```python
from build123d import *

# Parameters (mm, degrees)
F0_W     = 101.6
F0_H     = 101.6
F1_DEPTH = 6.35
F2_R     = 3.175
F3_DEPTH = 6.351
F4_W     = 6.35
F4_H     = 50.8
F5_DEPTH = 6.351


with BuildPart() as f1:
    # F0 (on Top) → F1 (new body)
    with BuildSketch(Plane.XY):
        Rectangle(F0_W, F0_H)
    extrude(amount=F1_DEPTH)

    # F2 (on Top) → F3 (cut, through all)
    with BuildSketch(Plane.XY):
        with Locations((-6.35, 0)):
            Circle(F2_R)
    extrude(amount=F3_DEPTH, mode=Mode.SUBTRACT)

    # F4 (on Top) → F5 (cut, through all)
    with BuildSketch(Plane.XY):
        with Locations((-41.275, 25.4)):
            Rectangle(F4_W, F4_H)
    extrude(amount=F5_DEPTH, mode=Mode.SUBTRACT)


solid = f1.part
```
Source: CAD feature listing. Evaluate the final solid. Frame: model axes, mm. A direction names the side the tool comes from. Round coordinates to 2 decimals unless told otherwise and drop trailing zeros. Loops run counter-clockwise (first coordinate to the right, second up) from the corner with the lowest first, then second, coordinate; pieces in that order, holes last.
1. Section query B-B on x = -6.35. Output: boundary loops of the cut face in (y, z) (3 decimals).
2. Ray query, L1, parallel to X at y = 43, z = 1.75; L2, parallel to Y at x = -6.35, z = 3 (3 decimals); L3, parallel to Y at x = -38.5, z = 3. Return the intervals inside material, ascending.
3. Section query C-C on z = 4.75. Output: boundary loops of the cut face in (x, y) (3 decimals).
4. Access query for faces 4 (the cylindrical face through (-3.32, 0.95, 3.13)), 5 (the flat face through (-41, 0, 3)). Directions: +Z, -Z, +X, -X, +Y, -Y. A direction counts if a zero-diameter tool reaches every point of the face in a straight line with its end or side. Return the directions, or none.
5. Contact query for a flat-ended pin moving along its axis: pin 1 (3 mm diameter, centred on x = -42, z = 4, fed in from +Y). Output: stop coordinate, or through.
6. Mould query, pull axis X, two halves, no side actions, for faces 1 (the flat face through (-44.45, 25, 3)), 2 (the flat face through (-50.8, -1, 3)), 3 (the flat face through (-1, -50.8, 3)). Classes: released by +X, released by -X, zero draft, split by the parting line, or undercut.
7. Section query A-A on y = 39. Output: boundary loops of the cut face in (x, z).
Answers below:
1. outline: (-50.8, 0) - (-3.175, 0) - (-3.175, 6.35) - (-50.8, 6.35) - close; (3.175, 0) - (50.8, 0) - (50.8, 6.35) - (3.175, 6.35) - close
2. L1: x = -50.8 to -44.45, -38.1 to 50.8
2. L2: y = -50.8 to -3.175, 3.175 to 50.8
2. L3: y = -50.8 to 0
3. outline: (-50.8, -50.8) - (50.8, -50.8) - (50.8, 50.8) - (-38.1, 50.8) - (-38.1, 0) - (-44.45, 0) - (-44.45, 50.8) - (-50.8, 50.8) - close; hole circle Ø6.35 at (-6.35, 0)
4. face 4: +Z, -Z
4. face 5: +Z, -Z, +Y
5. pin 1: stops at y = 0
6. face 1: undercut
6. face 2: released by -X
6. face 3: zero draft
7. outline: (-50.8, 0) - (-44.45, 0) - (-44.45, 6.35) - (-50.8, 6.35) - close; (-38.1, 0) - (50.8, 0) - (50.8, 6.35) - (-38.1, 6.35) - close
